The figure shows three views and two pictorial views of one solid part (mm, origin at its lowest corner). Answer the questions. Coordinates: 2 decimals unless noted, no trailing zeros. Order: outer loops, then holes, each group sorted by start corner. A loop starts at its lowest first (then second) coordinate and runs counter-clockwise, first axis right, second up. Notation, with made-up numbers: (84.5, 63) -> (123.5, 63) arc R19 cw to (123.5, 85) -> close; hole circle Ø7 at (-9, 24). An arc over 180 degrees is marked (long way). Write item = value, one per line. Start each with the question number.
Q1. The part is cut by section B-B, the plane z = 370. Determine the outline of the cut face in (x, y).
Q2. A flat-ended cylindrical pin translates along its axis: pin 1 (12 mm diameter, centred on y = 16.5, z = 372, fed in from -X). Find the tip coordinate at first contact, or state that the pin passes through.
Q3. Straight lines are drawn through the part: L1, parallel to Z at x = 262.5, y = 8.5; L2, parallel to Z at x = 115, y = 19.5; L3, parallel to X at y = 6.75, z = 360.5. For each, find the intervals that lie inside material, in ascending order. Write a range as from..to.
Q4. The part is cut by section C-C, the plane y = 15.5. Determine the outline of the cut face in (x, z).
Q5. The part is cut by section A-A, the plane x = 262.5. Determine the outline of the cut face in (y, z), plus the area to 3 significant figures.
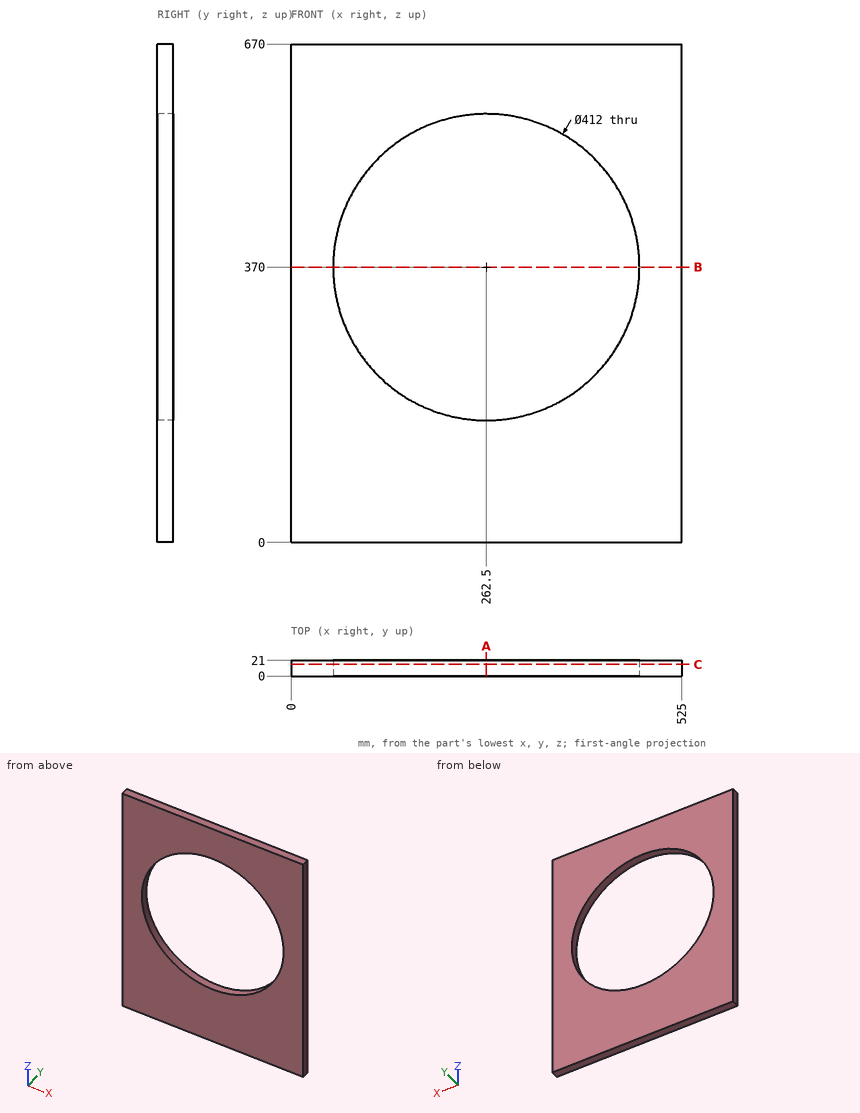
Model answer:
q1.outline = (0, 0) -> (56.5, 0) -> (56.5, 21) -> (0, 21) -> close; (468.5, 0) -> (525, 0) -> (525, 21) -> (468.5, 21) -> close
q2.pin_1 = 0
q3.L1 = 0..164, 576..670
q3.L2 = 0..226.2, 513.8..670
q3.L3 = 0..56.72, 468.28..525
q4.outline = (0, 0) -> (525, 0) -> (525, 670) -> (0, 670) -> close; hole circle Ø412 at (262.5, 370)
q5.outline = (0, 0) -> (21, 0) -> (21, 164) -> (0, 164) -> close; (0, 576) -> (21, 576) -> (21, 670) -> (0, 670) -> close
q5.area = 5,420 mm2
